The listing builds one solid part. Answer for the finished solid, in the listing's coordinates (mm). Coordinates: 2 decimals unless noted, no trailing zeros. Write item = value, one per line.
from build123d import *

# Parameters (mm, degrees)
SKETCH1_W           = 212
SKETCH1_H           = 153
SKETCH1_R           = 1.75
SKETCH1_R_2         = 2
BOSS_EXTRUDE1_DEPTH = 4
FILLET1_R           = 4


with BuildPart() as part:
    # Sketch1 → Boss-Extrude1 (new body)
    with BuildSketch(Plane.XY):
        Rectangle(SKETCH1_W, SKETCH1_H)
        with Locations((-96.5, -61)):
            Circle(SKETCH1_R, mode=Mode.SUBTRACT)
        with Locations(Location((-8.5, -61, 0), (0, 0, 180))):
            Circle(SKETCH1_R, mode=Mode.SUBTRACT)
        with Locations((8.5, -61)):
            Circle(SKETCH1_R, mode=Mode.SUBTRACT)
        with Locations(Location((96.5, -61, 0), (0, 0, 180))):
            Circle(SKETCH1_R, mode=Mode.SUBTRACT)
        with Locations(Location((-96.5, 67, 0), (0, 0, 180))):
            Circle(SKETCH1_R, mode=Mode.SUBTRACT)
        with Locations((96.5, 67)):
            Circle(SKETCH1_R, mode=Mode.SUBTRACT)
        with Locations(Location((8.5, 67, 0), (0, 0, 180))):
            Circle(SKETCH1_R, mode=Mode.SUBTRACT)
        with Locations((-8.5, 67)):
            Circle(SKETCH1_R, mode=Mode.SUBTRACT)
        with Locations((-96.5, -71)):
            Circle(SKETCH1_R_2, mode=Mode.SUBTRACT)
        with Locations(Location((95.480310976, -73.51, 0), (0, 0, 180))):
            Circle(SKETCH1_R_2, mode=Mode.SUBTRACT)
        with Locations((-64.5, -71)):
            Circle(SKETCH1_R_2, mode=Mode.SUBTRACT)
        with Locations((63.480310976, -73.51)):
            Circle(SKETCH1_R_2, mode=Mode.SUBTRACT)
    extrude(amount=BOSS_EXTRUDE1_DEPTH)

    # Fillet1
    fillet1_edges = [part.edges().sort_by_distance(p)[0] for p in [
        (-106, 76.5, 2),
        (106, 76.5, 2),
        (106, -76.5, 2),
        (-106, -76.5, 2),
    ]]
    fillet(fillet1_edges, radius=FILLET1_R)


solid = part.part
Q1. The mould has two halves that part along Y. Classify faces 1 (the face through (-106, -1, 2)), 2 (the face through (-95.425, -69.314, 1.972)), 3 (the face through (104.797, 75.359, 2.028)): released by +Y, released by -Y, zero draft, split by the parting line, or undercut.
The answers:
face_1 = zero draft
face_2 = undercut
face_3 = released by +Y
Q2. Find the intervals of material crossed by line 1 along Y through (x, z) = (-8.5, 0.8); line 2 along X through (y, z) = (-70, 0.85); line 3 along Y through (x, z) = (-63, 2.2), in increasing order.
The answers:
line_1 = -76.5 to -62.75, -59.25 to 65.25, 68.75 to 76.5
line_2 = -106 to -98.23, -94.77 to -66.23, -62.77 to 106
line_3 = -76.5 to -72.32, -69.68 to 76.5
Q3. Each of these flat-tipped pins is pushed along its axis until it touches: pin 1 Ø1.5 at (x, y) = (31.5, 20.5) entering from -Z; pin 2 Ø3 at (x, y) = (-96.5, 67) entering from -Z. Where does it stop, or does it pass through?
The answers:
pin_1 = 0
pin_2 = through
